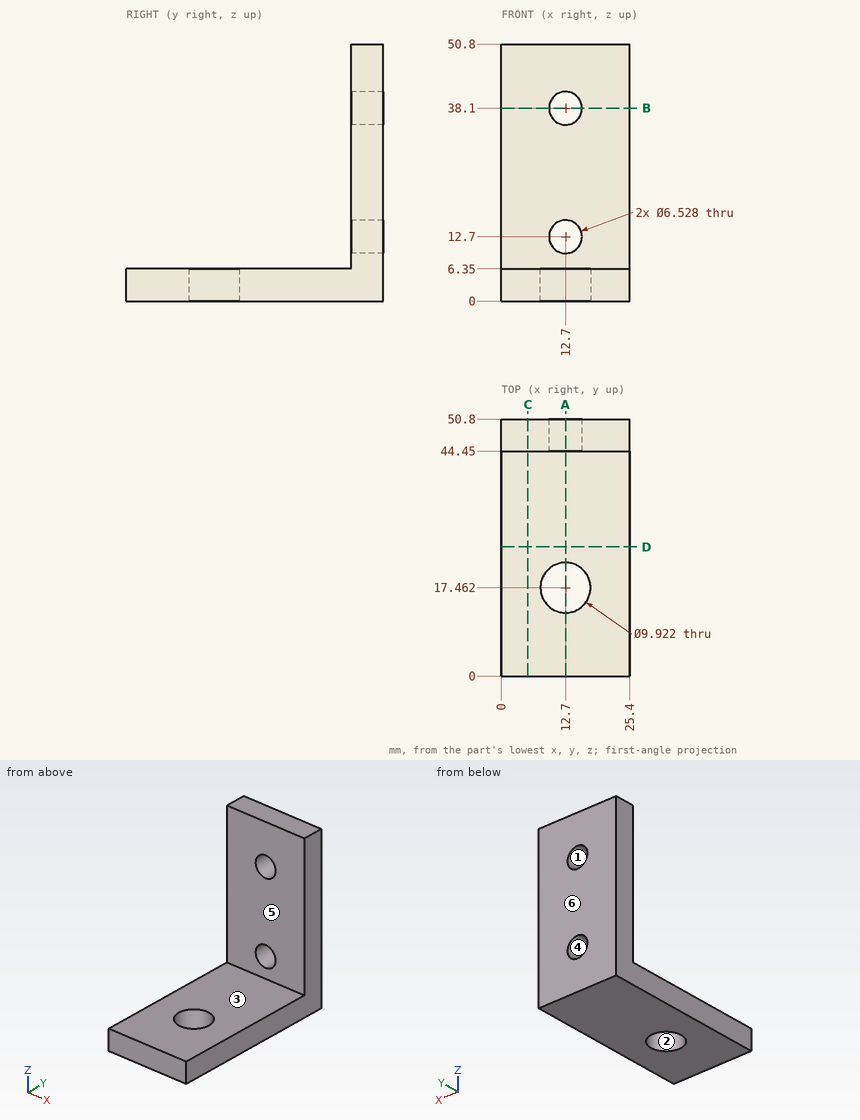
The figure shows three views and two pictorial views of one solid part (mm, origin at its lowest corner). Answer the questions. A direction names the side the tool comes from. Give positions to 0.01 mm unless a question says otherwise; leave off trailing zeros. Order: outer loops, then holes, each group sorted by start corner. A loop starts at its lowest first (then second) coordinate and runs counter-clockwise, first axis right, second up. Notation, with made-up numbers: M 89.25,33.25 L 142.25,33.25 A13 ccw 142.25,55.25 Z; hole C 89,86 d2. An arc over 180 degrees is marked long. Return JSON: item names as keys, results as strings.
Q1. The mould has two halves that part along Z. Classify the marked faces 1, 2, 3 and 4: pulls with the +Z half, pulls with the -Z half, needs draft (parallel to the pull), parting line crosses it, or undercut.
Answer below:
{"face 1": "undercut", "face 2": "needs draft", "face 3": "pulls with the +Z half", "face 4": "undercut"}
Q2. Find the intervals of material crossed by line 1 along Z through (x, y) = (12.7, 46.25); line 2 along Y through (x, z) = (12.7, 2.5); line 3 along Y through (x, z) = (7.5, 32.5), in increasing order. Write a range as [from, to].
Answer below:
{"line 1": "z = [0, 9.44], [15.96, 34.84], [41.36, 50.8]", "line 2": "y = [0, 12.5], [22.42, 50.8]", "line 3": "y = [44.45, 50.8]"}
Q3. Which of the six approach directions +Z, -Z, +X, -X, +Y, -Y give full straight-line access (tool end or side, diameter ignored) to the marked faces 5 and 6?
Answer below:
{"face 5": "+Z, +X, -X, -Y", "face 6": "+Z, -Z, +X, -X, +Y"}
Q4. Find section D-D, the plane y = 25.5. Write down the section's boundary in (x, z), and give its area (3 significant figures).
Answer below:
{"outline": "M 0,0 L 25.4,0 L 25.4,6.35 L 0,6.35 Z", "area": "161 mm^2"}
Q5. Find section A-A, the plane x = 12.7. Write down the section's boundary in (y, z).
Answer below:
{"outline": "M 0,0 L 12.5,0 L 12.5,6.35 L 0,6.35 Z; M 22.42,0 L 50.8,0 L 50.8,9.44 L 44.45,9.44 L 44.45,6.35 L 22.42,6.35 Z; M 44.45,15.96 L 50.8,15.96 L 50.8,34.84 L 44.45,34.84 Z; M 44.45,41.36 L 50.8,41.36 L 50.8,50.8 L 44.45,50.8 Z"}
Q6. Find section B-B, the plane z = 38.1. Write down the section's boundary in (x, y), and give its area (3 significant figures).
Answer below:
{"outline": "M 0,44.45 L 9.44,44.45 L 9.44,50.8 L 0,50.8 Z; M 15.96,44.45 L 25.4,44.45 L 25.4,50.8 L 15.96,50.8 Z", "area": "120 mm^2"}
Q7. Find section C-C, the plane x = 5.25. Write down the section's boundary in (y, z).
Answer below:
{"outline": "M 0,0 L 50.8,0 L 50.8,50.8 L 44.45,50.8 L 44.45,6.35 L 0,6.35 Z"}
Q8. Each of these flat-tipped pins is pushed along its axis until it touches: pin 1 (1.5 mm diameter, centred on x = 8.5, y = 13.5, fed in from -Z); pin 2 (5 mm diameter, centred on x = 5.5, z = 20, fed in from -Y); pin 3 (7.5 mm diameter, centred on x = 17.5, y = 31, fed in from +Z). Where does it stop, or does it pass through?
Answer below:
{"pin 1": "stops at z = 0", "pin 2": "stops at y = 44.45", "pin 3": "stops at z = 6.35"}
